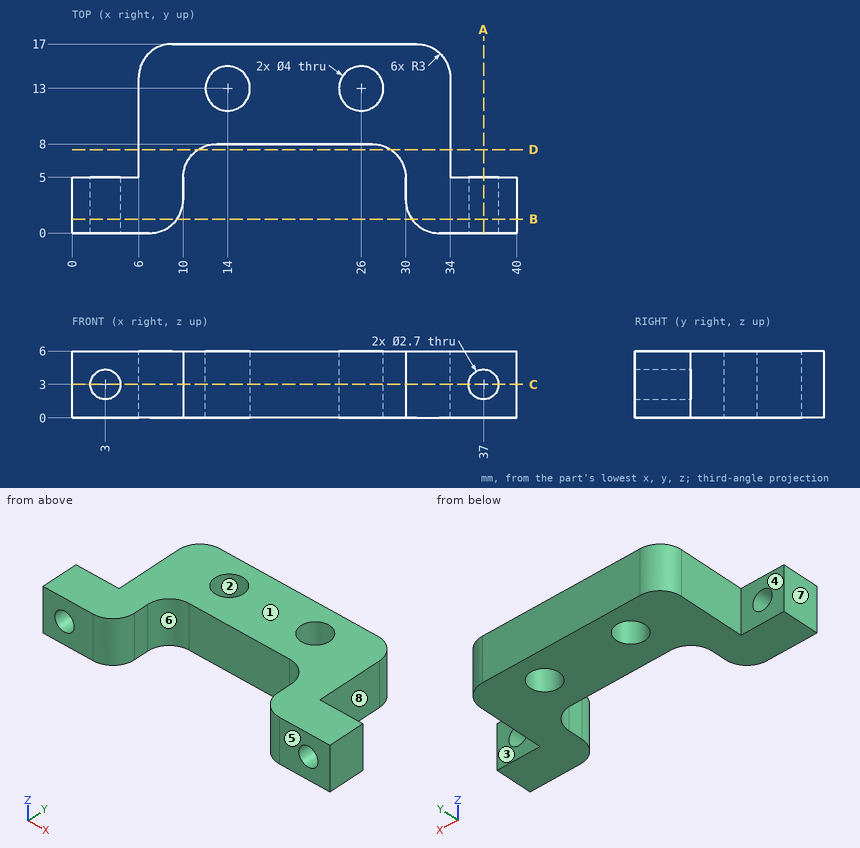
Geometry: see drawing. Coordinates: mm, zero at the bounding-box minimum. A direction names the side the tool comes from. Round coordinates to 2 decimals unless told otherwise and drop trailing zeros. Order: outer loops, then holes, each group sorted by start corner. A loop starts at its lowest first (then second) coordinate and runs counter-clockwise, first axis right, second up. Notation, with made-up numbers: (-8, 25) - (37, 25) arc R23 cw to (37, 43) - close; hole circle Ø10 at (31.5, 57.25). An arc over 180 degrees is marked (long way). Use a Markdown table: item, result. Add a question column.
1. Section query D-D (y = 7.5). Return the cut outline in (x, z), then the cut area to 3 significant figures.
2. Set-up query: the marked faces 4, 5, 6, 7 and 8. Return all of +Z, -Z, +X, -X, +Y, -Y with unobstructed straight access to the full face (end or side cutting, diameter ignored); none if empty.
3. Section query B-B (y = 1.25). Return the cut outline in (x, z), then the cut area to 3 significant figures.
4. Mould query, pull axis Y, two halves, no side actions, for the marked faces 1, 2 and 3. Classes: +Y half, -Y half, draft (parallel to the pull), parting line (faces both ways), or undercut.
5. Section query A-A (x = 37). Return the cut outline in (y, z), then the cut area to 3 significant figures.
6. First-contact query: pin 1 (3 mm diameter, centred on x = 37, z = 3, fed in from +Y); pin 2 (2 mm diameter, centred on y = 10.5, z = 4.5, fed in from -X); pin 3 (4 mm diameter, centred on x = 13.5, y = 4.5, fed in from +Z). Flat tips, straight axial feed; report the tip coordinate or a pass-through.
7. Line query: probe 1 along Y at (x, z) = (14, 4.6); probe 2 along X at (y, z) = (4, 1.4); probe 3 along X at (y, z) = (14.5, 1.65). Output: solid intervals per line, ascending.
8. Section query C-C (z = 3). Return the cut outline in (x, y), then the cut area to 3 significant figures.
Derived:
| question | item | result |
|---|---|---|
| 1 | outline | (6, 0) - (11.34, 0) - (11.34, 6) - (6, 6) - close; (28.66, 0) - (34, 0) - (34, 6) - (28.66, 6) - close |
| 1 | area | 64.1 mm2 |
| 2 | face 4 | +Z, -Z, -X, +Y |
| 2 | face 5 | +Z, -Z, +X, -X, -Y |
| 2 | face 6 | +Z, -Z, -Y |
| 2 | face 7 | +Z, -Z, -X, +Y, -Y |
| 2 | face 8 | +Z, -Z, +X, +Y |
| 3 | outline | (0, 0) - (9.44, 0) - (9.44, 6) - (0, 6) - close; (30.56, 0) - (40, 0) - (40, 6) - (30.56, 6) - close; hole circle Ø2.7 at (3, 3); hole circle Ø2.7 at (37, 3) |
| 3 | area | 102 mm2 |
| 4 | face 1 | draft |
| 4 | face 2 | undercut |
| 4 | face 3 | +Y half |
| 5 | outline | (0, 0) - (5, 0) - (5, 1.65) - (0, 1.65) - close; (0, 4.35) - (5, 4.35) - (5, 6) - (0, 6) - close |
| 5 | area | 16.5 mm2 |
| 6 | pin 1 | y = 5 |
| 6 | pin 2 | x = 6 |
| 6 | pin 3 | through |
| 7 | probe 1 | 8 to 11, 15 to 17 |
| 7 | probe 2 | 0 to 10, 30 to 40 |
| 7 | probe 3 | 6.04 to 12.68, 15.32 to 24.68, 27.32 to 33.96 |
| 8 | outline | (0, 0) - (1.65, 0) - (1.65, 5) - (0, 5) - close; (4.35, 0) - (7, 0) arc R3 ccw to (10, 3) - (10, 5) arc R3 cw to (13, 8) - (27, 8) arc R3 cw to (30, 5) - (30, 3) arc R3 ccw to (33, 0) - (35.65, 0) - (35.65, 5) - (34, 5) - (34, 14) arc R3 ccw to (31, 17) - (9, 17) arc R3 ccw to (6, 14) - (6, 5) - (4.35, 5) - close; (38.35, 0) - (40, 0) - (40, 5) - (38.35, 5) - close; hole circle Ø4 at (14, 13); hole circle Ø4 at (26, 13) |
| 8 | area | 320 mm2 |
